Autodesk Inventor part; units mm, degrees
ref_plane "YZ Plane" through (0, 0, 0) normal (1, 0, 0) x (0, 1, 0)
ref_plane "XZ Plane" through (0, 0, 0) normal (0, 1, 0) x (-1, 0, 0)
ref_plane "XY Plane" through (0, 0, 0) normal (0, 0, 1) x (1, 0, 0)
sketch "スケッチ1" plane through (0, 0, 0) normal (1, 0, 0) x (0, 1, 0)
  line L0 (5, 5) -> (-5, 5)
  line L1 (-5, 5) -> (-5, -5)
  line L2 (-5, -5) -> (5, -5)
  line L3 (5, -5) -> (5, 5)
  line L4 (4, 4) -> (-4, 4)
  line L5 (-4, 4) -> (-4, -4)
  line L6 (-4, -4) -> (4, -4)
  line L7 (4, -4) -> (4, 4)
  point P0 (0, 0)
  dimension "d0" = 1
  dimension "d1" = 1
  dimension "d2" = 1
  dimension "d3" = 1
  dimension "d4" = 10
  dimension "d5" = 10
  dimension "d6" = 5
  dimension "d7" = 5
extrude "押し出し1" add sketch "スケッチ1" along normal blind 50
sketch "スケッチ2" plane through (0, -5, 5) normal (0, 0, 1) x (1, 0, 0)
  circle A0 centre (15, 5) radius 1.5
  line L0 (0, 0) -> (50, 0)
  line L1 (0, 10) -> (0, 0)
  point P0 (0, 5)
  dimension "d10" = 5
  dimension "d11" = 3
  dimension "d12" = 15
extrude "押し出し2" cut sketch "スケッチ2" against normal blind 50
sketch "スケッチ3" plane through (0, -5, -5) normal (0, -1, 0) x (1, 0, 0)
  circle A0 centre (5, 5) radius 1.5
  line L0 (0, 10) -> (0, 0)
  line L1 (0, 0) -> (50, 0)
  point P0 (0, 5)
  dimension "d15" = 5
  dimension "d16" = 5
  dimension "d17" = 3
extrude "押し出し3" cut sketch "スケッチ3" against normal blind 50
sketch "スケッチ4" plane through (0, -5, -5) normal (0, 0, -1) x (-1, 0, 0)
  circle A0 centre (-45, 5) radius 1.5
  line L0 (0, 10) -> (-50, 10)
  line L1 (-50, 0) -> (-50, 10)
  point P0 (0, 5)
  dimension "d20" = 3
  dimension "d21" = 5
  dimension "d22" = 5
extrude "押し出し4" cut sketch "スケッチ4" against normal blind 50
properties part number "flontparts1" material "アルミニウム 6061"
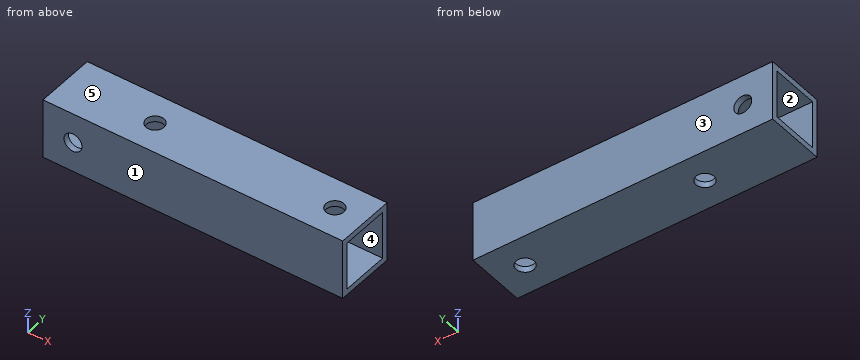
Read the model definition and answer for the solid it produces. Units are mm, in the model's axes. Face numbers are marked on the shaded views. A direction names the side the tool comes from. Coordinates: 2 decimals unless noted, no trailing zeros. Loops run counter-clockwise (first coordinate to the right, second up) from the corner with the lowest first, then second, coordinate; pieces in that order, holes last. Notation, with made-up numbers: (54.5, -28.75) -> (91.5, -28.75) arc R18 cw to (91.5, -16.75) -> close; hole circle Ø4 at (-32, 5). An arc over 180 degrees is marked (long way). Write item = value, one per line. Start each with the question number.
1) The part is cut by section C-C, the plane x = 5. Determine the outline of the cut face in (y, z).
2) Given P1, Ø3, axis at y = -1.5, z = 1, coming from the +X side, flat-ended and moving along its own axis, determine where the tip first touches the part or whether it passes through.
3) The part is cut by section A-A, the plane y = 2.75. Determine the outline of the cut face in (x, z), plus the area to 3 significant figures.
4) For the marked faces 4 and 5, determine the directions among +Z, -Z, +X, -X, +Y, -Y from which every point of the face is accessible in a straight line to the end or side of a thin tool.
5) The mould has two halves that part along Y. Classify the marked faces 1, 2 and 3: pulls with the +Y half, pulls with the -Y half, needs draft (parallel to the pull), parting line crosses it, or undercut.
6) The part is cut by section D-D, the plane z = 0. Determine the outline of the cut face in (x, y).
7) Find the intervals of material crossed by L1, parallel to Z at x = 6, y = -1; L2, parallel to Y at x = 45, z = 4.55; L3, parallel to X at y = 0.5, z = 4.25, in increasing order. Write a range as from..to.
Result:
q1.outline = (-5, -5) -> (5, -5) -> (5, -1.5) -> (4, -1.5) -> (4, -4) -> (-4, -4) -> (-4, -1.5) -> (-5, -1.5) -> close; (-5, 1.5) -> (-4, 1.5) -> (-4, 4) -> (4, 4) -> (4, 1.5) -> (5, 1.5) -> (5, 5) -> (-5, 5) -> close
q2.P1 = through
q3.outline = (0, -5) -> (50, -5) -> (50, -4) -> (0, -4) -> close; (0, 4) -> (50, 4) -> (50, 5) -> (0, 5) -> close
q3.area = 100 mm²
q4.face_4 = +X, -X
q4.face_5 = +Z, +X, -X, +Y, -Y
q5.face_1 = pulls with the -Y half
q5.face_2 = undercut
q5.face_3 = pulls with the +Y half
q6.outline = (0, -5) -> (3.5, -5) -> (3.5, -4) -> (0, -4) -> close; (0, 4) -> (3.5, 4) -> (3.5, 5) -> (0, 5) -> close; (6.5, -5) -> (50, -5) -> (50, -4) -> (6.5, -4) -> close; (6.5, 4) -> (50, 4) -> (50, 5) -> (6.5, 5) -> close
q7.L1 = -5..-4, 4..5
q7.L2 = -5..-1.5, 1.5..5
q7.L3 = 0..13.59, 16.41..43.59, 46.41..50
